Design review of the part built by this model. Coordinates are the model's own, in mm. A direction names the side the tool comes from. Round coordinates to 2 decimals unless told otherwise and drop trailing zeros. Order: outer loops, then holes, each group sorted by start corner. A loop starts at its lowest first (then second) coordinate and runs counter-clockwise, first axis right, second up. Notation, with made-up numbers: (19.25, 26) - (32.25, 26) arc R35 cw to (32.25, 60) - close; hole circle Ø1 at (82.25, 50). An arc over 180 degrees is marked (long way). Write item = value, one per line.
from build123d import *

# Parameters (mm, degrees)
SKETCH1_W           = 25
SKETCH1_H           = 3.5
BOSS_EXTRUDE1_DEPTH = 3.9
SKETCH1_3_W         = 12.4
SKETCH1_3_H         = 22.6
CUT_EXTRUDE3_DEPTH  = 4.9


with BuildPart() as part:
    # Sketch1 → Boss-Extrude1 (new body)
    with BuildSketch(Plane(origin=(0, 0, 0), x_dir=(1, 0, 0), z_dir=(0, 1, 0))):
        Polygon((-76.1, 25), (-100, 25), (-100, 10), (-96.1, 10), (-96.1, -10), (-100, -10), (-100, -25), (100, -25), (100, -10), (96.1, -10), (96.1, 10), (100, 10), (100, 25), (76.1, 25), (76.1, 28.9), (56.1, 28.9), (56.1, 25), (10, 25), (10, 28.9), (-10, 28.9), (-10, 25), (-56.1, 25), (-56.1, 28.9), (-76.1, 28.9), align=None)
        with Locations((-12.5, 11.85)):
            Rectangle(SKETCH1_W, SKETCH1_H, mode=Mode.SUBTRACT)
    extrude(amount=BOSS_EXTRUDE1_DEPTH)

    # Sketch1<3> → Cut-Extrude3 (cut, through all)
    with BuildSketch(Plane(origin=(0, 0, 0), x_dir=(1, 0, 0), z_dir=(0, 1, 0))):
        with Locations((0, -8.7)):
            Rectangle(SKETCH1_3_W, SKETCH1_3_H)
    extrude(amount=CUT_EXTRUDE3_DEPTH, mode=Mode.SUBTRACT)


solid = part.part
Item 1: Take a section at C-C, the plane y = 2.15. Count the separate pieces of the cut face and the enclosed holes in it, and give its area (3 significant figures).
Data:
separate_pieces = 1
enclosed_holes = 2
area = 9,710 mm2
Item 2: For line 1 along Z through (x, y) = (-0.5, 1.2); line 2 along X through (y, z) = (2.3, 4.5); line 3 along X through (y, z) = (3.25, -10.5), list the stretches that pass through material, from the lowest coordinate up. Write a range as [from, to].
Data:
line_1 = [-28.9, -13.6], [-10.1, -2.6], [20, 25]
line_2 = [-96.1, -6.2], [6.2, 96.1]
line_3 = [-100, -25], [0, 100]
Item 3: The part is to be moulded in two halves that separate along Z. For faces 1 (the face through (-1, 2, 25)), 2 (the face through (-96.1, 2, 0)), 3 (the face through (-100, 2, 17)), 4 (the face through (-33, 2, -25)), say which applies: +Z half, -Z half, draft (parallel to the pull), parting line (faces both ways), or undercut.
Data:
face_1 = +Z half
face_2 = undercut
face_3 = draft
face_4 = -Z half
Item 4: Take a section at D-D, the plane x = 29. State the section outline as (y, z) points, and give its area (3 significant figures).
Data:
outline = (0, -25) - (3.9, -25) - (3.9, 25) - (0, 25) - close
area = 195 mm2
Item 5: Insertion check: P1, Ø1.2, axis at x = 92, y = 2.5, coming from the -Z side; P2, Ø2, axis at y = 2.5, z = -3, coming from the -X side; P3, Ø1.9, axis at y = 1, z = -26.5, coming from the +X side. Each pin has a flat end and moves straight along its axis. Give the tip position at first contact, or say it passes through.
Data:
P1 = -25
P2 = -96.1
P3 = 76.1
Item 6: Take a section at A-A, the plane x = -20. State the section outline as (y, z) points.
Data:
outline = (0, -25) - (3.9, -25) - (3.9, -13.6) - (0, -13.6) - close; (0, -10.1) - (3.9, -10.1) - (3.9, 25) - (0, 25) - close
Item 7: Take a section at B-B, the plane z = 2. State the section outline as (x, y) points.
Data:
outline = (-96.1, 0) - (-6.2, 0) - (-6.2, 3.9) - (-96.1, 3.9) - close; (6.2, 0) - (96.1, 0) - (96.1, 3.9) - (6.2, 3.9) - close
Item 8: For faces 5 (the face through (-98, 2, 10)), 6 (the face through (-56.1, 2, -27)), 7 (the face through (76.1, 2, -27)), 8 (the face through (-76.1, 2, -27)), 9 (the face through (0, 2, -2.6)), list the 3-axis set-ups (+Z, -Z, +X, -X, +Y, -Y) from which the entire face can be reached by the end or side of a thin tool; tool diameter is ignored.
Data:
face_5 = -X, +Y, -Y
face_6 = -Z, +Y, -Y
face_7 = -Z, +X, +Y, -Y
face_8 = -Z, -X, +Y, -Y
face_9 = +Y, -Y
